Design review of the part shown in the three views and the two pictorial views. Dimensions are in mm from the part's minimum x, y and z. Round coordinates to 2 decimals unless told otherwise and drop trailing zeros. Loops run counter-clockwise (first coordinate to the right, second up) from the corner with the lowest first, then second, coordinate; pieces in that order, holes last. Notation, with made-up numbers: (-1, 39.25) - (55, 39.25) arc R19 cw to (55, 49.25) - close; hole circle Ø5 at (42.5, -2.75). An arc over 180 degrees is marked (long way). Return JSON: item names as keys, results as strings. Group by question number.
(1) Wall thickness on L1, parallel to X at y = 3.1, z = 1.05; L2, parallel to Z at x = 3.55, y = 2.35: over which ranges is each line inside the solid? List them lowest first. Write a range as [from, to].
(2) We need section B-B, the plane z = 1.2. Write out the cut boundary in (x, y), and give its area (3 significant figures).
(3) We need section A-A, the plane x = 4.1. Write out the cut boundary in (y, z), and give its area (3 significant figures).
(4) We need section C-C, the plane y = 4.35. Write out the cut boundary in (x, z), and give its area (3 significant figures).
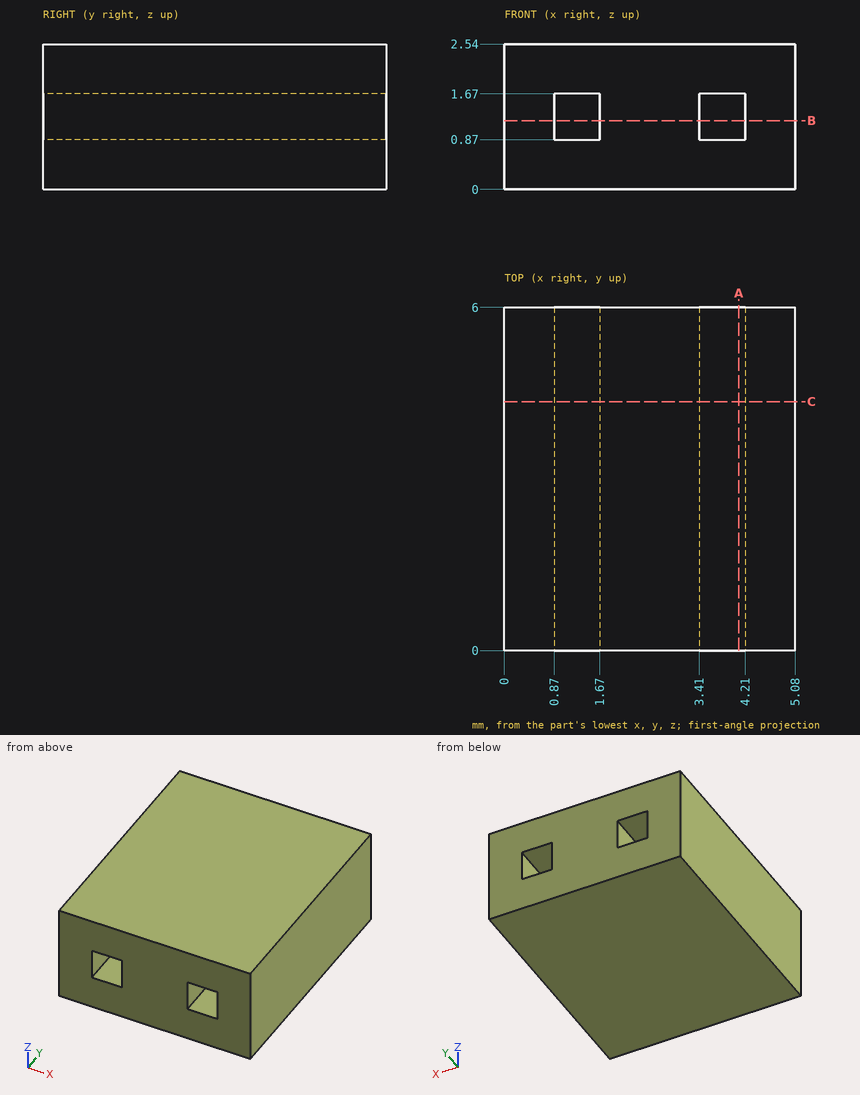
Solutions:
{
 "1": {"L1": "[0, 0.87], [1.67, 3.41], [4.21, 5.08]", "L2": "[0, 0.87], [1.67, 2.54]"},
 "2": {"outline": "(0, 0) - (0.87, 0) - (0.87, 6) - (0, 6) - close; (1.67, 0) - (3.41, 0) - (3.41, 6) - (1.67, 6) - close; (4.21, 0) - (5.08, 0) - (5.08, 6) - (4.21, 6) - close", "area": "20.9 mm^2"},
 "3": {"outline": "(0, 0) - (6, 0) - (6, 0.87) - (0, 0.87) - close; (0, 1.67) - (6, 1.67) - (6, 2.54) - (0, 2.54) - close", "area": "10.4 mm^2"},
 "4": {"outline": "(0, 0) - (5.08, 0) - (5.08, 2.54) - (0, 2.54) - close; hole (0.87, 0.87) - (1.67, 0.87) - (1.67, 1.67) - (0.87, 1.67) - close; hole (3.41, 0.87) - (4.21, 0.87) - (4.21, 1.67) - (3.41, 1.67) - close", "area": "11.6 mm^2"}
}
